```python
from build123d import *

# Parameters (mm, degrees)
BOSS_EXTRUDE1_DEPTH = 0.9525


with BuildPart() as part:
    # Sketch1 → Boss-Extrude1 (new, symmetric)
    with BuildSketch(Plane.XY):
        with BuildLine():
            Line((-5.715, 12.7), (5.715, 12.7))
            ThreePointArc((5.715, 12.7), (8.409076836, 11.584076836), (9.525, 8.89))
            Line((9.525, 8.89), (9.525, -8.89))
            ThreePointArc((9.525, -8.89), (8.409076836, -11.584076836), (5.715, -12.7))
            Line((5.715, -12.7), (-5.715, -12.7))
            ThreePointArc((-5.715, -12.7), (-8.409076836, -11.584076836), (-9.525, -8.89))
            Line((-9.525, -8.89), (-9.525, 8.89))
            ThreePointArc((-9.525, 8.89), (-8.409076836, 11.584076836), (-5.715, 12.7))
        make_face()
        Polygon((-3.85275, -6.367292239), (-3.85275, -7.874), (3.85275, -7.874), (3.85275, -6.367292239), (0.9, -6.367292239), (0.9, 6.367292239), (3.85275, 6.367292239), (3.85275, 7.874), (-3.85275, 7.874), (-3.85275, 6.367292239), (-0.9, 6.367292239), (-0.9, -6.367292239), align=None, mode=Mode.SUBTRACT)
    extrude(amount=BOSS_EXTRUDE1_DEPTH, both=True)


solid = part.part
```
The model under review builds one solid part; all positions refer to its coordinate system, in mm. A direction names the side the tool comes from. Round coordinates to 2 decimals unless told otherwise and drop trailing zeros. Order: outer loops, then holes, each group sorted by start corner. A loop starts at its lowest first (then second) coordinate and runs counter-clockwise, first axis right, second up. Notation, with made-up numbers: M 51,87 L 92,87 A11 ccw 92,93 Z; hole C 13.5,64 d11. An arc over 180 degrees is marked long. Use a Markdown table: item, result.
1) Draft analysis for pull direction Y (two halves, no side actions). For faces 1 (the face through (-3.853, -7, 0)), 2 (the face through (-8.44, 11.55, 0.01)), 3 (the face through (0, -7.874, 0)), 4 (the face through (9.525, 0, 0)), state which applies: released by +Y, released by -Y, zero draft, split by the parting line, or undercut.
Report:
| item | result |
|---|---|
| face 1 | undercut |
| face 2 | released by +Y |
| face 3 | undercut |
| face 4 | zero draft |
2) Consider section B-B (y = 0.25). Write out the cut boundary in (x, z) (1 decimal), then the cut area to 3 significant figures.
Report:
| item | result |
|---|---|
| outline | M -9.5,-1 L -0.9,-1 L -0.9,1 L -9.5,1 Z; M 0.9,-1 L 9.5,-1 L 9.5,1 L 0.9,1 Z |
| area | 32.9 mm^2 |
3) Wall thickness on line 1 along Y through (x, z) = (-3.75, 0.55); line 2 along X through (y, z) = (4.25, 0.4) (3 decimals); line 3 along X through (y, z) = (7.5, -0.7) (3 decimals): over which ranges is each line inside the solid? List them lowest first. Write a range as [from, to].
Report:
| item | result |
|---|---|
| line 1 | [-12.7, -7.87], [-6.37, 6.37], [7.87, 12.7] |
| line 2 | [-9.525, -0.9], [0.9, 9.525] |
| line 3 | [-9.525, -3.853], [3.853, 9.525] |
4) Consider section C-C (z = 0.6). Write out the cut boundary in (x, y) (3 decimals), then the cut area to 3 significant figures.
Report:
| item | result |
|---|---|
| outline | M -9.525,-8.89 A3.81 ccw -5.715,-12.7 L 5.715,-12.7 A3.81 ccw 9.525,-8.89 L 9.525,8.89 A3.81 ccw 5.715,12.7 L -5.715,12.7 A3.81 ccw -9.525,8.89 Z; hole M -3.853,-7.874 L 3.853,-7.874 L 3.853,-6.367 L 0.9,-6.367 L 0.9,6.367 L 3.853,6.367 L 3.853,7.874 L -3.853,7.874 L -3.853,6.367 L -0.9,6.367 L -0.9,-6.367 L -3.853,-6.367 Z |
| area | 425 mm^2 |
5) Consider section A-A (x = 0). Write out the cut boundary in (y, z).
Report:
| item | result |
|---|---|
| outline | M -12.7,-0.95 L -7.87,-0.95 L -7.87,0.95 L -12.7,0.95 Z; M 7.87,-0.95 L 12.7,-0.95 L 12.7,0.95 L 7.87,0.95 Z |
6) Consider section D-D (x = 7.75). Write out the cut boundary in (y, z).
Report:
| item | result |
|---|---|
| outline | M -12.11,-0.95 L 12.11,-0.95 L 12.11,0.95 L -12.11,0.95 Z |
7) Tool access review of faces 5 (the face through (0, -12.7, 0)), 6 (the face through (2, 6.367, 0)): name each direction out of +Z, -Z, +X, -X, +Y, -Y from which nothing blocks a thin tool from reaching the whole face with its end or side.
Report:
| item | result |
|---|---|
| face 5 | +Z, -Z, +X, -X, -Y |
| face 6 | +Z, -Z |
